Part model, mm, in its own coordinate system. Round coordinates to 2 decimals unless told otherwise and drop trailing zeros. Loops run counter-clockwise (first coordinate to the right, second up) from the corner with the lowest first, then second, coordinate; pieces in that order, holes last. Notation, with made-up numbers: (31.25, 72.25) -> (36.25, 72.25) arc R26 cw to (36.25, 108.25) -> close; hole circle Ø11 at (-15, 15). An arc over 180 degrees is marked (long way). Answer as CSV lines item,"result".
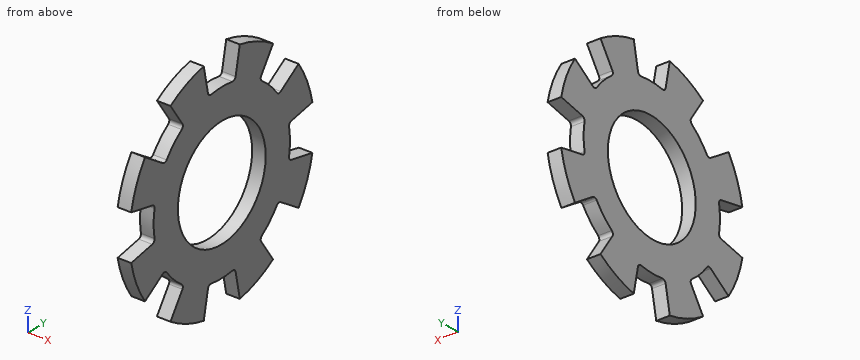
Autodesk Inventor part; units mm, degrees
ref_plane "Work Plane1" through (0, 0, 0) normal (0, -1, 0) x (1, 0, 0)
ref_plane "YZ Plane" through (0, 0, 0) normal (1, 0, 0) x (0, 1, 0)
ref_plane "XZ Plane" through (0, 0, 0) normal (0, 1, 0) x (-1, 0, 0)
sketch "Sketch1" plane through (0, 0, 0) normal (1, 0, 0) x (0, 1, 0)
  circle A0 centre (0, 0) radius 5.207
  circle A1 centre (0, 0) radius 2.4765
  dimension "d0" = 10.414
  dimension "d1" = 4.953
extrude "Body" add sketch "Sketch1" along normal blind 0.6096
sketch "Sketch2" plane through (0.6096, 0, 0) normal (1, 0, 0) x (0, 0, -1)
  circle A0 centre (0, 0) radius 5.207
  line L0 (0, 0) -> (0, 5.207) construction
  arc A1 (1.0158, 5.1069) -> (-1.0158, 5.1069) centre (0, 0) ccw
  arc A2 (0.7495, 3.7679) -> (-0.7495, 3.7679) centre (0, 0) ccw
  line L1 (-0.7495, 3.7679) -> (-1.0158, 5.1069)
  line L2 (0.7495, 3.7679) -> (1.0158, 5.1069)
  line L3 (-0.7495, 3.7679) -> (0, 0) construction
  line L4 (0, 0) -> (0.7495, 3.7679) construction
  dimension "d4" = 22.5
  dimension "d5" = 7.6835
extrude "Cut" cut sketch "Sketch2" against normal through all contours L2 A2 L1 A0 picked at (-0.0838, 4.7417)
fillet "Fillet1" radius 0.1562 2 edges at (0.3048, 3.7679, 0.7495) (0.3048, 3.7679, -0.7495)
pattern_circular "Cuts" count 8 over 360 about axis through (0, 0, 0) along (1, 0, 0) of "Cut", "Fillet1"
ref_plane "Work Plane1" through (0, 0, 0) normal (0, -1, 0) x (1, 0, 0)
equation "\"d0\" = SD2"
equation "\"d1\" = SD1"
equation "\"d2\" = SD"
equation "\"d5\" = 0.5 * SD2 + 0.5 * SD1"
equation "\"d6\" = SD"
equation "\"d8\" = 0.015 * SD2"
equation "\"SD\" = 0.6096"
equation "\"SD1\" = 4.953"
equation "\"SD2\" = 10.414"
equation "\"NND\" = 4.826"
properties part number "ASME B18.21.1 - No. 10. Carbon Steel"
Q1. Drop a flat-ended pin along its axis: P1, Ø2, axis at y = -1, z = -0.5, coming from the -X side. Give the stop position or say it passes through.
Geometry results:
P1,"through"
Q2. Drill centre lines: line 1 along Z through (x, y) = (0.45, 0); line 2 along Y through (x, z) = (0.1, 2.25); line 3 along Y through (x, z) = (0.1, 2.75). Where is each one in solid material? Low to high.
Geometry results:
line 1,"-3.84 to -2.48, 2.48 to 3.84"
line 2,"-4.7 to -3.37, -3.11 to -1.03, 1.03 to 3.11, 3.37 to 4.7"
line 3,"-4.42 to -4.12, -2.68 to 2.68, 4.12 to 4.42"
Q3. Saw through at A-A, the plane y = 0. Write the cut outline in (x, z).
Geometry results:
outline,"(0, -3.84) -> (0.61, -3.84) -> (0.61, -2.48) -> (0, -2.48) -> close; (0, 2.48) -> (0.61, 2.48) -> (0.61, 3.84) -> (0, 3.84) -> close"
Q4. Saw through at C-C, the plane y = 3.5. Write the cut outline in (x, z), then the cut area to 3 significant figures.
Geometry results:
outline,"(0, -2.34) -> (0.61, -2.34) -> (0.61, 2.34) -> (0, 2.34) -> close"
area,"2.85 mm2"
